Geometry check sheet. Reference: the model listing, model coordinates, mm. A direction names the side the tool comes from. Coordinates: 2 decimals unless noted, no trailing zeros. Loops run counter-clockwise (first coordinate to the right, second up) from the corner with the lowest first, then second, coordinate; pieces in that order, holes last. Notation, with made-up numbers: (83.25, 19) - (122.25, 19) arc R24 ccw to (122.25, 34) - close; hole circle Ø10 at (82, -14.5). An arc over 180 degrees is marked (long way). Write each question's results on one line, items separated by ' | '. Start each with the question number.
(1) Sectioned sample at A-A (y = 0). Enter the section's corners in (x, z), plus the area to 3 significant figures.
(2) Mould release check, pull along Z, two halves, no side actions. Record for faces 1 (the face through (139.87, -72.69, 70.16)), 2 (the face through (331, -76.2, 39)), 3 (the face through (-14.88, -2.134, 392.727)): pulls with the +Z half, pulls with the -Z half, needs draft (parallel to the pull), parting line crosses it, or undercut.
(3) Sectioned sample at D-D (y = 118). Enter the section's corners in (x, z), plus the area to 3 significant figures.
(4) Access from +Z, -Z, +X, -X, +Y, -Y to the whole of each face (thin tool, end or side, straight path). Record for faces 4 (the face through (-63, 25.4, 134)), 5 (the face through (64, 25.4, 134)), 6 (the face through (-25.4, -63, 121)), 7 (the face through (-331, -76.2, 39)), 8 (the face through (329, 76.2, 39)).
(5) Sectioned sample at B-B (z = 246.5). Enter the section's corners in (x, y).
(6) Material ranges on probe 1 along Y at (x, z) = (-152, 55); probe 2 along X at (y, z) = (-78, 28); probe 3 along X at (y, z) = (-17, 279), recorded low to high.
(7) Go/stop test with flat-tipped pins: pin 1 Ø10 at (y, z) = (-2, 80.5) entering from -X; pin 2 Ø1 at (x, y) = (30.5, 77.5) entering from +Z; pin 3 Ø6 at (x, z) = (-3.5, 162) entering from +Y; pin 4 Ø23 at (x, y) = (152.4, -76.2) entering from -Z. Record where each tip stops, or that it passes through.
(8) Sectioned sample at C-C (x = 213). Enter the section's corners in (y, z), plus the area to 3 significant figures.
from build123d import *

# Parameters (mm, degrees)
F0_W            = 762
F0_H            = 304.8
F1_DEPTH        = 76.2
F3_DEPTH        = 203.2
F4_R            = 114.3
F4_R_2          = 76.2
F5_DEPTH        = 152.4
F6_DEPTH        = 152.4
F8_R            = 76.2
F10_DEPTH       = 76.201
F11_D           = 25.4
F11_CSINK_D     = 38.1
F11_CSINK_ANGLE = 90


# Not quite as in the source:
# - a pattern or mirror of a feature is missing from the dataset's text; its kind, count and spacing are read off the source's solid


with BuildPart() as f1:
    # F0 (on Top) → F1 (new body)
    with BuildSketch(Plane.XY):
        Rectangle(F0_W, F0_H)
    extrude(amount=F1_DEPTH)

    # F2 (on face) → F3 (join)
    with BuildSketch(Plane.XY.offset(76.2)):
        Polygon((101.6, -25.4), (101.6, 25.4), (25.4, 25.4), (25.4, 101.6), (-25.4, 101.6), (-25.4, 25.4), (-101.6, 25.4), (-101.6, -25.4), (-25.4, -25.4), (-25.4, -101.6), (25.4, -101.6), (25.4, -25.4), align=None)
    extrude(amount=F3_DEPTH)

    # F4 (on Front) → F5 (join, symmetric)
    with BuildSketch(Plane.XZ):
        with Locations((0, 279.4)):
            Circle(F4_R)
        with Locations((0, 279.4)):
            Circle(F4_R_2, mode=Mode.SUBTRACT)
    extrude(amount=F5_DEPTH, both=True)

    # F4 (on Front) → F6 (cut, symmetric)
    with BuildSketch(Plane.XZ):
        with Locations((0, 279.4)):
            Circle(F4_R_2)
    extrude(amount=F6_DEPTH, both=True, mode=Mode.SUBTRACT)

    # F8
    f8_edges = [f1.edges().sort_by_distance(p)[0] for p in [
        (381, 152.4, 38.1),
        (-381, 152.4, 38.1),
        (381, -152.4, 38.1),
        (-381, -152.4, 38.1),
    ]]
    fillet(f8_edges, radius=F8_R)

    # F9 (on face) → F10 (cut, through all)
    with BuildSketch(Plane.XY.offset(76.2)):
        with BuildLine():
            Line((-381, -76.2), (-279.4, -76.2))
            ThreePointArc((-279.4, -76.2), (-203.2, 0), (-279.4, 76.2))
            Line((-279.4, 76.2), (-381, 76.2))
            Line((-381, 76.2), (-381, -76.2))
        make_face()
    f10 = extrude(amount=-F10_DEPTH, mode=Mode.SUBTRACT)

    # F10_copies: F10 across plane
    add(f10.mirror(Plane(origin=(0, 0, 0), x_dir=(0, 0, 1), z_dir=(1, 0, 0))), mode=Mode.SUBTRACT)

    # F11 (through all)
    with Locations(Plane.XY.offset(76.2)):
        with Locations((-152.4, 76.2)):
            f11 = CounterSinkHole(F11_D / 2, F11_CSINK_D / 2, counter_sink_angle=F11_CSINK_ANGLE)

    # F11_copies: F11 across plane
    add(f11.mirror(Plane(origin=(0, 0, 0), x_dir=(0, 0, -1), z_dir=(0, -1, 0))), mode=Mode.SUBTRACT)

    # F11_copies1: F11 across plane
    add(f11.mirror(Plane(origin=(0, 0, 0), x_dir=(0, 0, 1), z_dir=(1, 0, 0))), mode=Mode.SUBTRACT)

    # F11_copies2: F11 across plane
    add(f11.mirror(Plane(origin=(0, 0, 0), x_dir=(0.4472135955, 0.894427191, 0), z_dir=(0.894427191, -0.4472135955, 0))), mode=Mode.SUBTRACT)


solid = f1.part
Outcome:
1) outline: (-203.2, 0) - (203.2, 0) - (203.2, 76.2) - (101.6, 76.2) - (101.6, 227.04) arc R114.3 ccw (long way) to (-101.6, 227.04) - (-101.6, 76.2) - (-203.2, 76.2) - close; hole circle Ø152.4 at (0, 279.4) | area: 75,400 mm2
2) face 1: pulls with the +Z half | face 2: needs draft | face 3: undercut
3) outline: (-368.51, 0) - (368.51, 0) - (368.51, 76.2) - (-368.51, 76.2) - close; circle Ø228.6 at (0, 279.4); hole circle Ø152.4 at (0, 279.4) | area: 79,000 mm2
4) face 4: -X, +Y | face 5: +X, +Y | face 6: -X, -Y | face 7: +Z, -Z, -X | face 8: +Z, -Z, +X
5) outline: (-109.46, -152.4) - (-68.73, -152.4) - (-68.73, 152.4) - (-109.46, 152.4) - close; (68.73, -152.4) - (109.46, -152.4) - (109.46, 152.4) - (68.73, 152.4) - close
6) probe 1: y = -152.4 to -88.89, -63.51 to 63.51, 88.89 to 152.4 | probe 2: x = -380.98 to -164.97, -139.83 to 139.83, 164.97 to 380.98 | probe 3: x = -114.3 to -76.2, 76.2 to 114.3
7) pin 1: stops at x = -203.34 | pin 2: stops at z = 389.69 | pin 3: stops at y = 101.6 | pin 4: passes through
8) outline: (-152.4, 0) - (-37.38, 0) - (-37.38, 76.2) - (-152.4, 76.2) - close; (37.38, 0) - (152.4, 0) - (152.4, 76.2) - (37.38, 76.2) - close | area: 17,500 mm2
